```python
from build123d import *

# Parameters (mm, degrees)
BASE_DEPTH              = 13
SKETCH2_R               = 1.4
SCREW_HOLES_DEPTH       = 63.860957676
F_8MM_BRACKET_FILLETS_R = 8
F_1MM_EDGE_FILLETS_R    = 1


with BuildPart() as part:
    # Sketch1 → Base (new, symmetric)
    with BuildSketch(Plane(origin=(0, 0, 0), x_dir=(0, 0, -1), z_dir=(1, 0, 0))):
        Polygon((0, 27.25), (0, 21.25), (-22.5, 21.25), (-22.5, -21.25), (0, -21.25), (0, -27.25), (-28.5, -27.25), (-28.5, 27.25), align=None)
    extrude(amount=BASE_DEPTH, both=True)

    # Sketch2 → Screw Holes (cut, through all)
    with BuildSketch(Plane(origin=(0, 27.25, 0), x_dir=(1, 0, 0), z_dir=(0, 1, 0))):
        with Locations(Location((-8, -5, 0), (0, 0, 270))):
            Circle(SKETCH2_R)
        with Locations(Location((8, -5, 0), (0, 0, 270))):
            Circle(SKETCH2_R)
    extrude(amount=-SCREW_HOLES_DEPTH, mode=Mode.SUBTRACT)

    # 8mm Bracket Fillets
    f_8mm_bracket_fillets_edges = [part.edges().sort_by_distance(p)[0] for p in [
        (0, 21.25, 22.5),
        (0, -21.25, 22.5),
        (0, -27.25, 28.5),
        (0, 27.25, 28.5),
    ]]
    fillet(f_8mm_bracket_fillets_edges, radius=F_8MM_BRACKET_FILLETS_R)

    # 1mm Edge Fillets
    f_1mm_edge_fillets_edges = [part.edges().sort_by_distance(p)[0] for p in [
        (-13, 27.25, 10.25),
        (13, -21.25, 7.25),
        (-13, 21.25, 7.25),
        (13, 21.25, 7.25),
        (-13, 0, 22.5),
        (13, 0, 22.5),
        (-13, 0, 28.5),
        (13, 0, 28.5),
        (-13, -27.25, 10.25),
        (-13, -24.906854249, 26.156854249),
        (13, 27.25, 10.25),
        (-13, 24.906854249, 26.156854249),
        (13, -27.25, 10.25),
        (13, -24.906854249, 26.156854249),
        (13, 24.906854249, 26.156854249),
        (-13, 18.906854249, 20.156854249),
        (13, 18.906854249, 20.156854249),
        (-13, -18.906854249, 20.156854249),
        (13, -18.906854249, 20.156854249),
        (-13, -21.25, 7.25),
    ]]
    fillet(f_1mm_edge_fillets_edges, radius=F_1MM_EDGE_FILLETS_R)


solid = part.part
```
Read the model definition and answer for the solid it produces. Units are mm, in the model's axes. A direction names the side the tool comes from. Give positions to 0.01 mm unless a question says otherwise; leave off trailing zeros. Order: outer loops, then holes, each group sorted by start corner. A loop starts at its lowest first (then second) coordinate and runs counter-clockwise, first axis right, second up.
(1) Find section B-B (x = 8). Give the vertices of the cut face in (y, z).
(2) For a pull along Z with two mould halves and no side action, classify faces 1 (the flat face through (0, 0, 22.5)), 2 (the flat face through (0, 21.25, 7)), 3 (the cylindrical face through (-9.24, -24.21, 5.65)) as released by +Z, released by -Z, zero draft, split by the parting line, or undercut.
(3) Given pin 1 (3 mm diameter, centred on x = -5, y = 17, fed in from -Z); pin 2 (6 mm diameter, centred on x = -8, y = -7, fed in from -Z), each flat-ended and moving along its own axis, determine where each tip first touches the part or whether it passes through.
(4) Find section A-A (z = 5). Give the number of separate pieces and of enclosed holes in the cut face, plus the area to 3 significant figures.
(5) Find section C-C (z = 13.25). Give the vertices of the cut face in (x, y).
(6) For faces 4 (the cylindrical face through (7.46, 24.29, 6.29)), 5 (the flat face through (0, -21.25, 7)), determine the directions among +Z, -Z, +X, -X, +Y, -Y from which every point of the face is accessible in a straight line to the end or side of a thin tool.
(7) Straight lines are drawn through the part: L1, parallel to X at y = 22.5, z = 5; L2, parallel to Y at x = 0, z = 7; L3, parallel to Y at x = 3.5, z = 19.25. For each, find the intervals that lie inside material, in ascending order.
(8) Find section D-D (y = -2.5). Give the vertices of the cut face in (x, z).
Result sheet:
1. outline: (-27.25, 0) - (-21.25, 0) - (-21.25, 3.6) - (-27.25, 3.6) - close; (-27.25, 6.4) - (-21.25, 6.4) - (-21.25, 14.5) arc R8 cw to (-13.25, 22.5) - (13.25, 22.5) arc R8 cw to (21.25, 14.5) - (21.25, 6.4) - (27.25, 6.4) - (27.25, 20.5) arc R8 ccw to (19.25, 28.5) - (-19.25, 28.5) arc R8 ccw to (-27.25, 20.5) - close; (21.25, 0) - (27.25, 0) - (27.25, 3.6) - (21.25, 3.6) - close
2. face 1: released by -Z
2. face 2: zero draft
2. face 3: undercut
3. pin 1: stops at z = 20.54
3. pin 2: stops at z = 22.5
4. separate pieces: 6
4. enclosed holes: 0
4. area: 243 mm2
5. outline: (-13, -26.25) arc R1 ccw to (-12, -27.25) - (12, -27.25) arc R1 ccw to (13, -26.25) - (13, -22.25) arc R1 ccw to (12, -21.25) - (-12, -21.25) arc R1 ccw to (-13, -22.25) - close; (-13, 22.25) arc R1 ccw to (-12, 21.25) - (12, 21.25) arc R1 ccw to (13, 22.25) - (13, 26.25) arc R1 ccw to (12, 27.25) - (-12, 27.25) arc R1 ccw to (-13, 26.25) - close
6. face 4: +Y, -Y
6. face 5: -Z, +X, -X
7. L1: x = -13 to -9.4, -6.6 to 6.6, 9.4 to 13
7. L2: y = -27.25 to -21.25, 21.25 to 27.25
7. L3: y = -27.25 to -19.69, 19.69 to 27.25
8. outline: (-13, 23.5) arc R1 ccw to (-12, 22.5) - (12, 22.5) arc R1 ccw to (13, 23.5) - (13, 27.5) arc R1 ccw to (12, 28.5) - (-12, 28.5) arc R1 ccw to (-13, 27.5) - close
